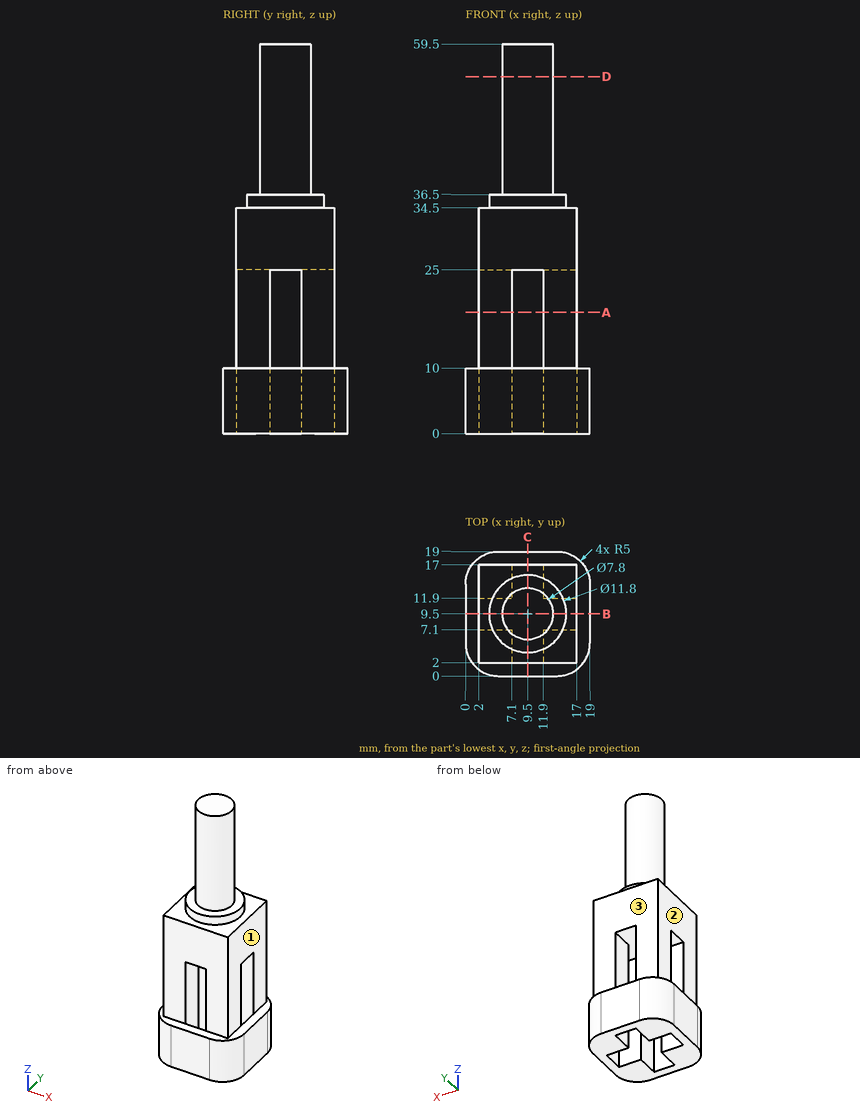
Input: dimensioned drawing with shaded views. Units: mm. Origin: part minimum x, y, z. A direction names the side the tool comes from. Coordinates: 2 decimals unless noted, no trailing zeros. Write each loop counter-clockwise with the first axis right and the second up, starting at its lowest first coordinate (ties: lowest second). Pieces come first, ordered by that corner, then holes. Notation, with made-up numbers: (14.5, -33.75) -> (31.5, -33.75) arc R19 ccw to (31.5, -20.75) -> close; hole circle Ø10 at (18, -36). An arc over 180 degrees is marked (long way). Return JSON: item names as keys, results as strings. Group by question number.
1) Set-up query: the marked faces 1, 2 and 3. Return all of +Z, -Z, +X, -X, +Y, -Y with unobstructed straight access to the full face (end or side cutting, diameter ignored); none if empty.
2) Section query A-A, the plane z = 18.5. Return loops of the section in (x, y).
3) Contact query for flat-ended pins moving along their axis: P1, Ø7.5, axis at y = 11, z = 23.5, coming from the -X side; P2, Ø1.5, axis at x = 13.5, z = 12.5, coming from the -Y side; P3, Ø1, axis at y = 7.5, z = 36, coming from the +X side; P4, Ø6, axis at x = 5, y = 16.5, coming from the -Z side. Output: stop coordinate, or through.
4) Section query D-D, the plane z = 54.5. Return loops of the section in (x, y).
5) Ray query, line 1 along Y through (x, z) = (14.25, 21); line 2 along Z through (x, y) = (1, 12). Return the intervals inside material, ascending.
6) Section query B-B, the plane y = 9.5. Return loops of the section in (x, z), plus the area to 4 significant figures.
From the geometry:
{
 "1": {"face 1": "+Z, +X, +Y, -Y", "face 2": "+Z, -X, +Y, -Y", "face 3": "+Z, +X, -X, +Y"},
 "2": {"outline": "(2, 2) -> (7.1, 2) -> (7.1, 7.1) -> (2, 7.1) -> close; (2, 11.9) -> (7.1, 11.9) -> (7.1, 17) -> (2, 17) -> close; (11.9, 2) -> (17, 2) -> (17, 7.1) -> (11.9, 7.1) -> close; (11.9, 11.9) -> (17, 11.9) -> (17, 17) -> (11.9, 17) -> close"},
 "3": {"P1": "x = 2", "P2": "y = 2", "P3": "x = 15.21", "P4": "z = 0"},
 "4": {"outline": "circle Ø7.8 at (9.5, 9.5)"},
 "5": {"line 1": "2 to 7.1, 11.9 to 17", "line 2": "0 to 10"},
 "6": {"outline": "(0, 0) -> (2, 0) -> (2, 10) -> (0, 10) -> close; (2, 25) -> (17, 25) -> (17, 34.5) -> (15.4, 34.5) -> (15.4, 36.5) -> (13.4, 36.5) -> (13.4, 59.5) -> (5.6, 59.5) -> (5.6, 36.5) -> (3.6, 36.5) -> (3.6, 34.5) -> (2, 34.5) -> close; (17, 0) -> (19, 0) -> (19, 10) -> (17, 10) -> close", "area": "385.5 mm²"}
}
